Part print with two shaded views. Sizes in mm from the minimum x, y, z corner. A direction names the side the tool comes from. Coordinates: 2 decimals unless noted, no trailing zeros. Order: outer loops, then holes, each group sorted by start corner. A loop starts at its lowest first (then second) coordinate and runs counter-clockwise, first axis right, second up. Notation, with made-up numbers: M 86,-8.5 L 125,-8.5 A14 ccw 125,3.5 Z; hole C -24,-40 d1. An arc over 180 degrees is marked long. Answer in a Markdown table with one row per item. Add a question column.
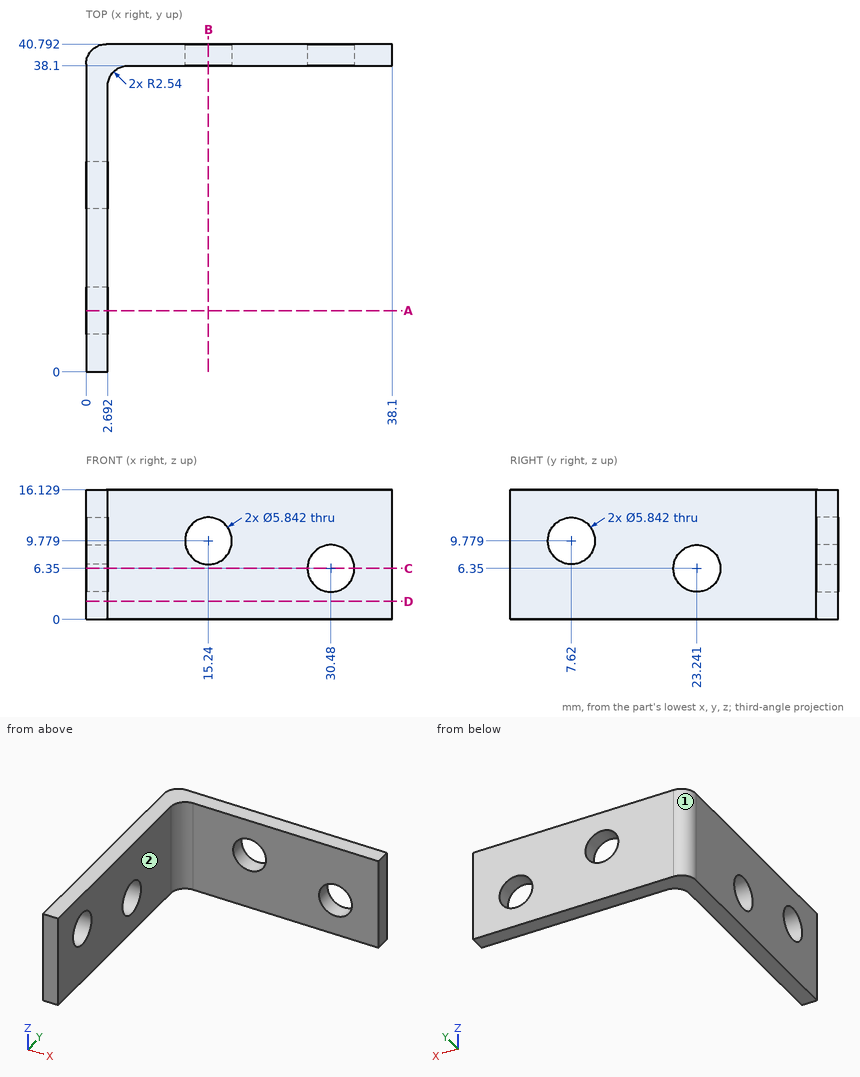
(1) Slice it at B-B (x = 15.24). List the corners of the cut face in (y, z), and give its area (3 significant figures).
(2) Wall check: line 1 (Y direction, x = 32, z = 14); line 2 (X direction, y = 13.5, z = 6.75); line 3 (X direction, y = 39.5, z = 6.35). Give the ranges that are in metal, low to high.
(3) Slice it at D-D (z = 2.25). List the corners of the cut face in (x, y), and give its area (3 significant figures).
(4) Drop flat-ended pins along their axis: P1, Ø8, axis at y = 15, z = 7, coming from the +X side; P2, Ø4.5, axis at x = 30.48, z = 6.35, coming from the +Y side (1 decimal); P3, Ø5, axis at x = 22, z = 10.5, coming from the -Y side. Give the stop position or say it passes through.
(5) Slice it at A-A (y = 7.62). List the corners of the cut face in (x, z).
(6) Slice it at C-C (z = 6.35). List the corners of the cut face in (x, y), and give its area (3 significant figures).
(7) 3-axis set-ups, long thin cutter, end or side, ignore diameter. For the marked faces 1 and 2: which of +Z, -Z, +X, -X, +Y, -Y reach the whole face in a straight line?
Computed:
| question | item | result |
|---|---|---|
| 1 | outline | M 38.1,0 L 40.79,0 L 40.79,6.86 L 38.1,6.86 Z; M 38.1,12.7 L 40.79,12.7 L 40.79,16.13 L 38.1,16.13 Z |
| 1 | area | 27.7 mm^2 |
| 2 | line 1 | y = 38.1 to 40.79 |
| 2 | line 2 | x = 0 to 2.69 |
| 2 | line 3 | x = 0.33 to 27.56, 33.4 to 38.1 |
| 3 | outline | M 0,0 L 2.69,0 L 2.69,35.56 A2.54 cw 5.23,38.1 L 38.1,38.1 L 38.1,40.79 L 2.54,40.79 A2.54 ccw 0,38.25 Z |
| 3 | area | 205 mm^2 |
| 4 | P1 | stops at x = 2.69 |
| 4 | P2 | passes through |
| 4 | P3 | stops at y = 38.1 |
| 5 | outline | M 0,0 L 2.69,0 L 2.69,6.86 L 0,6.86 Z; M 0,12.7 L 2.69,12.7 L 2.69,16.13 L 0,16.13 Z |
| 6 | outline | M 0,0 L 2.69,0 L 2.69,20.32 L 0,20.32 Z; M 0,26.16 L 2.69,26.16 L 2.69,35.56 A2.54 cw 5.23,38.1 L 27.56,38.1 L 27.56,40.79 L 2.54,40.79 A2.54 ccw 0,38.25 Z; M 33.4,38.1 L 38.1,38.1 L 38.1,40.79 L 33.4,40.79 Z |
| 6 | area | 174 mm^2 |
| 7 | face 1 | +Z, -Z, -X, +Y |
| 7 | face 2 | +Z, -Z, +X, -Y |
